For this review, take the finished solid that the model builds, in its own axes (mm). Face numbers are marked on the shaded views. Give positions to 0.01 mm unless a question says otherwise; leave off trailing zeros.
Item 1: The part is to be moulded in two halves that separate along Y. For the marked faces 1, 2, 3 and 4, say which applies: released by +Y, released by -Y, zero draft, split by the parting line, or undercut.
Item 2: For P1, Ø5, axis at y = 82.55, z = -6.35, coming from the +X side; P2, Ø12, axis at y = -22, z = 1, coming from the +X side (3 decimals); P3, Ø3, axis at x = -2.5, y = -65.5, coming from the +Z side, all flat-tipped, find the tip position at first contact; note any pin that passes through.
Item 3: Consider section A-A (x = -4.25). Give the number of separate pieces and of enclosed holes in the cut face, plus the area to 3 significant figures.
Item 4: For probe 1 along Z at (x, y) = (0.5, -88.9); probe 2 along Y at (x, z) = (3, -6); probe 3 along Y at (x, z) = (-2, -7.5), list the stretches that pass through material, from the lowest coordinate up.
```python
from build123d import *

# Parameters (mm, degrees)
F0_W     = 12.7
F0_H     = 25.4
F1_DEPTH = 101.6
F2_R     = 6.34999
F3_R     = 1.5875
F4_DEPTH = 25.4
F5_W     = 3.81
F5_H     = 107.95
F6_DEPTH = 25.4


# Not quite as in the source:
# - a fillet or chamfer is up to 0.001 mm smaller than in the source, because OpenCascade refuses the exact size


with BuildPart() as f1:
    # F0 (on Front) → F1 (new body, symmetric)
    with BuildSketch(Plane.XZ):
        Rectangle(F0_W, F0_H)
    extrude(amount=F1_DEPTH, both=True)

    # F2 (radius 6.35 in the source; OpenCascade refuses exactly that, so slightly less here)
    f2_edges = [f1.edges().sort_by_distance(p)[0] for p in [
        (-6.35, 0, 12.7),
        (6.35, 0, 12.7),
    ]]
    fillet(f2_edges, radius=F2_R)

    # F3 (on face) → F4 (cut)
    with BuildSketch(Plane(origin=(-6.35, 0, 0), x_dir=(0, -1, 0), z_dir=(-1, 0, 0))):
        with BuildLine():
            Line((-77.7875, 0), (-74.6125, 0))
            ThreePointArc((-74.6125, 0), (-76.2, 1.5875), (-77.7875, 0))
        make_face()
        with Locations((-88.9, 0)):
            Circle(F3_R)
        with BuildLine():
            ThreePointArc((90.4875, 0), (88.9, 1.5875), (87.3125, 0))
            ThreePointArc((87.3125, 0), (88.9, -1.5875), (90.4875, 0))
        make_face()
        with BuildLine():
            ThreePointArc((77.7875, 0), (76.2, 1.5875), (74.6125, 0))
            Line((74.6125, 0), (77.7875, 0))
        make_face()
        with BuildLine():
            Line((77.7875, 0), (74.6125, 0))
            ThreePointArc((74.6125, 0), (76.2, -1.5875), (77.7875, 0))
        make_face()
        with BuildLine():
            ThreePointArc((-77.7875, 0), (-76.2, -1.5875), (-74.6125, 0))
            Line((-74.6125, 0), (-77.7875, 0))
        make_face()
        with Locations((-82.55, -6.35)):
            Circle(F3_R)
        with Locations((82.55, -6.35)):
            Circle(F3_R)
    extrude(amount=-F4_DEPTH, mode=Mode.SUBTRACT)

    # F5 (on face) → F6 (cut)
    with BuildSketch(Plane(origin=(0, 0, -12.7), x_dir=(1, 0, 0), z_dir=(0, 0, -1))):
        with Locations((6.35, 0)):
            Rectangle(F5_W, F5_H)
    extrude(amount=-F6_DEPTH, mode=Mode.SUBTRACT)


solid = f1.part
```
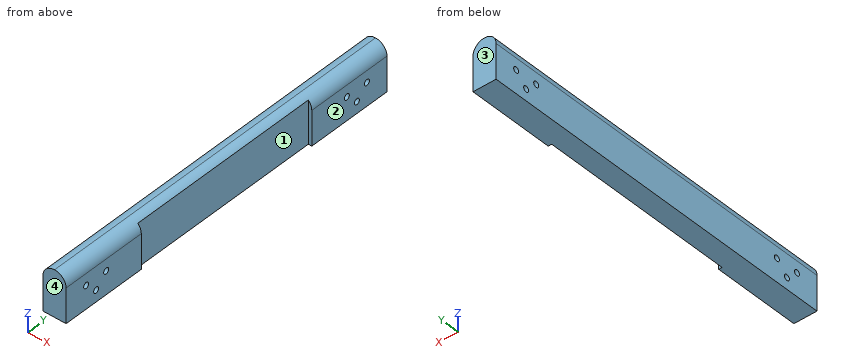
Resolved:
1. face 1: undercut
1. face 2: zero draft
1. face 3: released by +Y
1. face 4: released by -Y
2. P1: stops at x = 6.35
2. P2: stops at x = 4.445
2. P3: stops at z = 12.62
3. separate pieces: 1
3. enclosed holes: 6
3. area: 4,780 mm2
4. probe 1: z = -12.7 to -1.59, 1.59 to 12.68
4. probe 2: y = -101.6 to -84.1, -81 to 81, 84.1 to 101.6
4. probe 3: y = -101.6 to -83.64, -81.46 to 81.46, 83.64 to 101.6
